Geometry check sheet. Reference: the model listing, model coordinates, mm. Round coordinates to 2 decimals unless told otherwise and drop trailing zeros. Use a Markdown table: item, result.
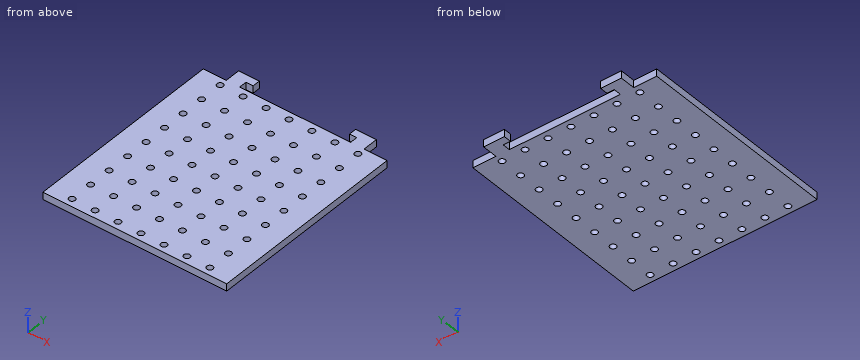
```python
from build123d import *

# Parameters (mm, degrees)
BOSS_EXTRUDE2_DEPTH     = 5.9944
F_1_4_20_TAPPED_HOLE1_D = 5.1054
FILL_START              = -5.9944
FILL_PATTERN1_OUTLINE_R = 2.5527
FILL_PATTERN1_DEPTH     = 5.9944


# Read off the part's stored shape, not the designer's step: Fill Pattern1
with BuildPart() as part:
    # Sketch1 → Boss-Extrude2 (new body)
    with BuildSketch(Plane.XY):
        Polygon((0, 0), (152.4, 0), (152.4, 165.1), (133.35, 165.1), (133.35, 177.8), (116.205, 177.8), (116.205, 171.45), (122.1994, 171.45), (122.1994, 165.1), (30.2006, 165.1), (30.2006, 171.45), (36.195, 171.45), (36.195, 177.8), (19.05, 177.8), (19.05, 165.1), (0, 165.1), align=None)
    extrude(amount=-BOSS_EXTRUDE2_DEPTH)

    # 1/4-20 Tapped Hole1 (through all)
    with Locations(Plane.XY):
        with Locations((76.2, 82.55)):
            Hole(F_1_4_20_TAPPED_HOLE1_D / 2)

    # Fill Pattern1 outline → Fill Pattern1 (cut)
    with BuildSketch(Plane.XY.offset(FILL_START)):
        with Locations((95.25, 63.5)):
            Circle(FILL_PATTERN1_OUTLINE_R)
        with Locations((76.2, 63.5)):
            Circle(FILL_PATTERN1_OUTLINE_R)
        with Locations((57.15, 63.5)):
            Circle(FILL_PATTERN1_OUTLINE_R)
        with Locations((57.15, 82.55)):
            Circle(FILL_PATTERN1_OUTLINE_R)
        with Locations((57.15, 101.6)):
            Circle(FILL_PATTERN1_OUTLINE_R)
        with Locations((76.2, 101.6)):
            Circle(FILL_PATTERN1_OUTLINE_R)
        with Locations((95.25, 101.6)):
            Circle(FILL_PATTERN1_OUTLINE_R)
        with Locations((95.25, 82.55)):
            Circle(FILL_PATTERN1_OUTLINE_R)
        with Locations((114.3, 44.45)):
            Circle(FILL_PATTERN1_OUTLINE_R)
        with Locations((95.25, 44.45)):
            Circle(FILL_PATTERN1_OUTLINE_R)
        with Locations((76.2, 44.45)):
            Circle(FILL_PATTERN1_OUTLINE_R)
        with Locations((57.15, 44.45)):
            Circle(FILL_PATTERN1_OUTLINE_R)
        with Locations((38.1, 44.45)):
            Circle(FILL_PATTERN1_OUTLINE_R)
        with Locations((38.1, 63.5)):
            Circle(FILL_PATTERN1_OUTLINE_R)
        with Locations((38.1, 82.55)):
            Circle(FILL_PATTERN1_OUTLINE_R)
        with Locations((38.1, 101.6)):
            Circle(FILL_PATTERN1_OUTLINE_R)
        with Locations((38.1, 120.65)):
            Circle(FILL_PATTERN1_OUTLINE_R)
        with Locations((57.15, 120.65)):
            Circle(FILL_PATTERN1_OUTLINE_R)
        with Locations((76.2, 120.65)):
            Circle(FILL_PATTERN1_OUTLINE_R)
        with Locations((95.25, 120.65)):
            Circle(FILL_PATTERN1_OUTLINE_R)
        with Locations((114.3, 120.65)):
            Circle(FILL_PATTERN1_OUTLINE_R)
        with Locations((114.3, 101.6)):
            Circle(FILL_PATTERN1_OUTLINE_R)
        with Locations((114.3, 82.55)):
            Circle(FILL_PATTERN1_OUTLINE_R)
        with Locations((114.3, 63.5)):
            Circle(FILL_PATTERN1_OUTLINE_R)
        with Locations((133.35, 25.4)):
            Circle(FILL_PATTERN1_OUTLINE_R)
        with Locations((114.3, 25.4)):
            Circle(FILL_PATTERN1_OUTLINE_R)
        with Locations((95.25, 25.4)):
            Circle(FILL_PATTERN1_OUTLINE_R)
        with Locations((76.2, 25.4)):
            Circle(FILL_PATTERN1_OUTLINE_R)
        with Locations((57.15, 25.4)):
            Circle(FILL_PATTERN1_OUTLINE_R)
        with Locations((38.1, 25.4)):
            Circle(FILL_PATTERN1_OUTLINE_R)
        with Locations((19.05, 25.4)):
            Circle(FILL_PATTERN1_OUTLINE_R)
        with Locations((19.05, 44.45)):
            Circle(FILL_PATTERN1_OUTLINE_R)
        with Locations((19.05, 63.5)):
            Circle(FILL_PATTERN1_OUTLINE_R)
        with Locations((19.05, 82.55)):
            Circle(FILL_PATTERN1_OUTLINE_R)
        with Locations((19.05, 101.6)):
            Circle(FILL_PATTERN1_OUTLINE_R)
        with Locations((19.05, 120.65)):
            Circle(FILL_PATTERN1_OUTLINE_R)
        with Locations((19.05, 139.7)):
            Circle(FILL_PATTERN1_OUTLINE_R)
        with Locations((38.1, 139.7)):
            Circle(FILL_PATTERN1_OUTLINE_R)
        with Locations((57.15, 139.7)):
            Circle(FILL_PATTERN1_OUTLINE_R)
        with Locations((76.2, 139.7)):
            Circle(FILL_PATTERN1_OUTLINE_R)
        with Locations((95.25, 139.7)):
            Circle(FILL_PATTERN1_OUTLINE_R)
        with Locations((114.3, 139.7)):
            Circle(FILL_PATTERN1_OUTLINE_R)
        with Locations((133.35, 139.7)):
            Circle(FILL_PATTERN1_OUTLINE_R)
        with Locations((133.35, 120.65)):
            Circle(FILL_PATTERN1_OUTLINE_R)
        with Locations((133.35, 101.6)):
            Circle(FILL_PATTERN1_OUTLINE_R)
        with Locations((133.35, 82.55)):
            Circle(FILL_PATTERN1_OUTLINE_R)
        with Locations((133.35, 63.5)):
            Circle(FILL_PATTERN1_OUTLINE_R)
        with Locations((133.35, 44.45)):
            Circle(FILL_PATTERN1_OUTLINE_R)
        with Locations((133.35, 6.35)):
            Circle(FILL_PATTERN1_OUTLINE_R)
        with Locations((114.3, 6.35)):
            Circle(FILL_PATTERN1_OUTLINE_R)
        with Locations((95.25, 6.35)):
            Circle(FILL_PATTERN1_OUTLINE_R)
        with Locations((76.2, 6.35)):
            Circle(FILL_PATTERN1_OUTLINE_R)
        with Locations((57.15, 6.35)):
            Circle(FILL_PATTERN1_OUTLINE_R)
        with Locations((38.1, 6.35)):
            Circle(FILL_PATTERN1_OUTLINE_R)
        with Locations((19.05, 6.35)):
            Circle(FILL_PATTERN1_OUTLINE_R)
        with Locations((19.05, 158.75)):
            Circle(FILL_PATTERN1_OUTLINE_R)
        with Locations((38.1, 158.75)):
            Circle(FILL_PATTERN1_OUTLINE_R)
        with Locations((57.15, 158.75)):
            Circle(FILL_PATTERN1_OUTLINE_R)
        with Locations((76.2, 158.75)):
            Circle(FILL_PATTERN1_OUTLINE_R)
        with Locations((95.25, 158.75)):
            Circle(FILL_PATTERN1_OUTLINE_R)
        with Locations((114.3, 158.75)):
            Circle(FILL_PATTERN1_OUTLINE_R)
        with Locations((133.35, 158.75)):
            Circle(FILL_PATTERN1_OUTLINE_R)
    extrude(amount=FILL_PATTERN1_DEPTH, mode=Mode.SUBTRACT)


solid = part.part
```
Item 1: Go/stop test with flat-tipped pins: pin 1 (6 mm diameter, centred on x = 53.5, y = 89, fed in from +Z); pin 2 (1.8 mm diameter, centred on x = 7, z = -2.5, fed in from +Y); pin 3 (1.8 mm diameter, centred on y = 169.5, z = -3, fed in from +X); pin 4 (1.8 mm diameter, centred on y = 171.5, z = -2.5, fed in from -X). Record where each tip stops, or that it passes through.
Outcome:
| item | result |
|---|---|
| pin 1 | stops at z = 0 |
| pin 2 | stops at y = 165.1 |
| pin 3 | stops at x = 133.35 |
| pin 4 | stops at x = 19.05 |
Item 2: Cross-section at A-A, the plane y = 158.75. Count the separate pieces of the cut face and the enclosed holes in it, and give its area (3 significant figures).
Outcome:
| item | result |
|---|---|
| separate pieces | 8 |
| enclosed holes | 0 |
| area | 699 mm2 |
Item 3: Material ranges on line 1 along X through (y, z) = (167, -1.05); line 2 along Y through (x, z) = (119, -1.8); line 3 along Y through (x, z) = (104, -4.75), recorded low to high. Write a range as from..to.
Outcome:
| item | result |
|---|---|
| line 1 | x = 19.05..30.2, 122.2..133.35 |
| line 2 | y = 0..165.1, 171.45..177.8 |
| line 3 | y = 0..165.1 |
